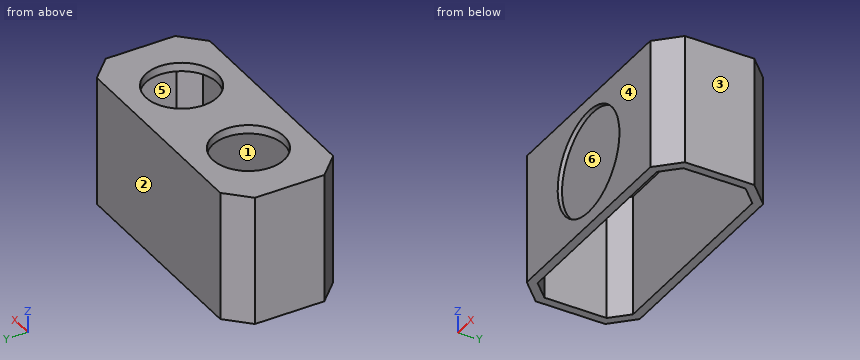
from build123d import *

# Parameters (mm, degrees)
SKETCH1_W          = 58
SKETCH1_H          = 26
SKULL_BLOCK_DEPTH  = 30
SKULL_CHAMFER_SIZE = 5
HOLLOW_SKULL_T     = -2
EYE_HOLE_REACH     = 45.704
SKETCH2_R          = 8.25
SKETCH3_R          = 12
NECK_MOUNT_DEPTH   = 1


with BuildPart() as part:
    # Sketch1 → skull block (new body)
    with BuildSketch(Plane.XY):
        Rectangle(SKETCH1_W, SKETCH1_H)
    extrude(amount=-SKULL_BLOCK_DEPTH)

    # skull chamfer
    skull_chamfer_edges = [part.edges().sort_by_distance(p)[0] for p in [
        (29, -13, -15),
        (-29, -13, -15),
        (-29, 13, -15),
        (29, 13, -15),
    ]]
    chamfer(skull_chamfer_edges, length=SKULL_CHAMFER_SIZE)

    # hollow skull
    hollow_skull_openings = [part.faces().sort_by_distance(p)[0] for p in [
        (0, 0, -30),
    ]]
    offset(amount=HOLLOW_SKULL_T, openings=hollow_skull_openings, kind=Kind.INTERSECTION)

    # Sketch2 → eye hole (cut, up to next)
    with BuildSketch(Plane.XY, mode=Mode.PRIVATE) as eye_hole_sk1:
        with Locations((13, 0)):
            Circle(SKETCH2_R)
    eye_hole_tool1 = extrude(eye_hole_sk1.sketch, amount=-EYE_HOLE_REACH, mode=Mode.PRIVATE) & part.part
    eye_hole = eye_hole_tool1.solids().sort_by_distance((13, 0, 0))[0]
    add(eye_hole, mode=Mode.SUBTRACT)

    # mirror eye hole: eye hole across plane
    add(eye_hole.mirror(Plane(origin=(0, 0, 0), x_dir=(0, 0, 1), z_dir=(1, 0, 0))), mode=Mode.SUBTRACT)

    # Sketch3 → neck mount (cut)
    with BuildSketch(Plane.XZ.offset(13)):
        with Locations(Location((0, -15, 0), (0, 0, 270))):
            Circle(SKETCH3_R)
    extrude(amount=-NECK_MOUNT_DEPTH, mode=Mode.SUBTRACT)


solid = part.part
Read the model definition and answer for the solid it produces. Units are mm, in the model's axes. Face numbers are marked on the shaded views. A direction names the side the tool comes from. Give positions to 0.01 mm unless a question says otherwise; leave off trailing zeros. Write each loop counter-clockwise with the first axis right and the second up, starting at its lowest first coordinate (ties: lowest second). Pieces come first, ordered by that corner, then holes. Notation, with made-up numbers: M 78.5,-23 L 114.5,-23 A28 cw 114.5,-3 Z; hole C -26,46 d6. An arc over 180 degrees is marked long. One line per item, written item: value. Start each with the question number.
(1) Find section C-C (y = 0). Determine the outline of the cut face in (x, z).
(2) Find section D-D (x = 0). Determine the outline of the cut face in (y, z), plus the area to 3 significant figures.
(3) A tool of negligible diameter and unlimited length cuts with its end or side. For the marked faces 4, 5 and 6, from which of +Z, -Z, +X, -X, +Y, -Y can it reach the whole face along a straight path? Write none if from no direction.
(4) Find section A-A (z = -15). Determine the outline of the cut face in (x, y).
(5) Determine the mould class of the marked faces 1, 2 and 3 for opening direction Y: pulls with the +Y half, pulls with the -Y half, needs draft (parallel to the pull), parting line crosses it, or undercut.
(6) A flat-ended cylindrical pin translates along its axis: pin 1 Ø1.5 at (x, y) = (10, 5.5) entering from -Z. Find the tip coordinate at first contact, or state that the pin passes through.
(7) Find section B-B (x = -13). Determine the outline of the cut face in (y, z), plus the area to 3 significant figures.
(8) Find the intervals of material crossed by line 1 (Y direction, x = -1, z = -18); line 2 (Y direction, x = 12, z = -25); line 3 (X direction, y = 6.25, z = -22.5), in increasing order.
Results below:
1. outline: M -29,-30 L -27,-30 L -27,-2 L -21.25,-2 L -21.25,0 L -29,0 Z; M -4.75,-2 L 4.75,-2 L 4.75,0 L -4.75,0 Z; M 21.25,-2 L 27,-2 L 27,-30 L 29,-30 L 29,0 L 21.25,0 Z
2. outline: M -13,-30 L -11,-30 L -11,-2 L 11,-2 L 11,-30 L 13,-30 L 13,0 L -13,0 L -13,-3 L -12,-3 L -12,-27 L -13,-27 Z
2. area: 140 mm^2
3. face 4: +Z, -Z, +X, -X, -Y
3. face 5: -Z
3. face 6: -Y
4. outline: M -29,-8 L -24,-13 L -12,-13 L -12,-12 L 12,-12 L 12,-13 L 24,-13 L 29,-8 L 29,8 L 24,13 L -24,13 L -29,8 Z; hole M -27,-7.17 L -23.17,-11 L 23.17,-11 L 27,-7.17 L 27,7.17 L 23.17,11 L -23.17,11 L -27,7.17 Z
5. face 1: undercut
5. face 2: pulls with the +Y half
5. face 3: needs draft
6. pin 1: passes through
7. outline: M -13,-30 L -11,-30 L -11,-2 L -8.25,-2 L -8.25,0 L -13,0 Z; M 8.25,-2 L 11,-2 L 11,-30 L 13,-30 L 13,0 L 8.25,0 Z
7. area: 131 mm^2
8. line 1: y = -12 to -11, 11 to 13
8. line 2: y = -13 to -11, 11 to 13
8. line 3: x = -29 to -27, 27 to 29
